Read the model definition and answer for the solid it produces. Units are mm, in the model's axes. Round coordinates to 2 decimals unless told otherwise and drop trailing zeros. Loops run counter-clockwise (first coordinate to the right, second up) from the corner with the lowest first, then second, coordinate; pieces in that order, holes last. Notation, with made-up numbers: M 69,-23.75 L 121,-23.75 A22 ccw 121,-14.75 Z; hole C 83.25,19 d9. An arc over 180 degrees is marked long. Answer as CSV lines item,"result".
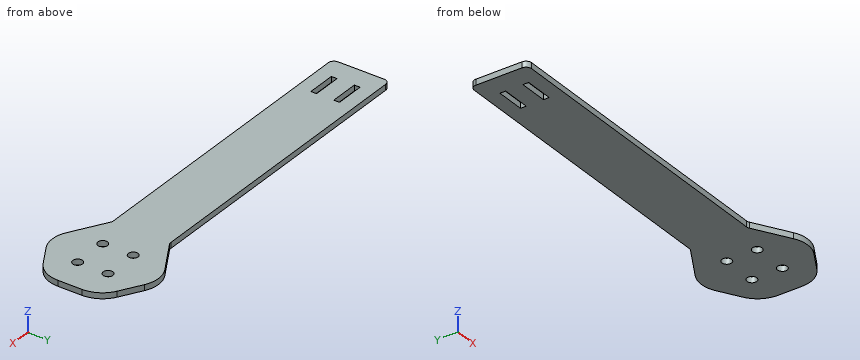
```python
from build123d import *

# Parameters (mm, degrees)
SKETCH1_W           = 107.330973451
SKETCH1_H           = 20
SKETCH1_W_2         = 10
SKETCH1_H_2         = 2
SKETCH1_R           = 12.25
SKETCH1_R_2         = 1.7
BOSS_EXTRUDE3_DEPTH = 2
FILLET5_R           = 10
FILLET6_R           = 10
FILLET7_R           = 10
FILLET8_R           = 10
FILLET14_R          = 2
FILLET15_R          = 2
FILLET16_R          = 2


with BuildPart() as part:
    # Sketch1 → Boss-Extrude3 (new body)
    # profile 1 of 4: a face of its own
    with BuildSketch(Plane.XY):
        with Locations((53.665486726, -20)):
            Rectangle(SKETCH1_W, SKETCH1_H)
        with Locations((12.5, -24)):
            Rectangle(SKETCH1_W_2, SKETCH1_H_2, mode=Mode.SUBTRACT)
        with Locations((12.5, -16)):
            Rectangle(SKETCH1_W_2, SKETCH1_H_2, mode=Mode.SUBTRACT)
    # profile 2 of 4: a face of its own
    with BuildSketch(Plane.XY):
        Polygon((140, -8.861471272), (124.651481526, 0), (107.330973451, -10), (107.330973451, -30), (124.651481526, -40), (140, -31.138528728), align=None)
        with Locations((124.651481526, -20)):
            Circle(SKETCH1_R, mode=Mode.SUBTRACT)
    # profile 3 of 4: a face of its own
    with BuildSketch(Plane.XY):
        with Locations((124.651481526, -20)):
            Circle(SKETCH1_R)
        with Locations((118.526481526, -25.304405598)):
            Circle(SKETCH1_R_2, mode=Mode.SUBTRACT)
        with Locations((130.776481526, -25.304405598)):
            Circle(SKETCH1_R_2, mode=Mode.SUBTRACT)
        with Locations((130.776481526, -14.695594402)):
            Circle(SKETCH1_R_2, mode=Mode.SUBTRACT)
        with Locations((118.526481526, -14.695594402)):
            Circle(SKETCH1_R_2, mode=Mode.SUBTRACT)
    # profile 4 of 4: a face of its own
    with BuildSketch(Plane.XY):
        Polygon((141.971989602, -10), (140, -8.861471272), (140, -31.138528728), (141.971989602, -30), align=None)
    extrude(amount=BOSS_EXTRUDE3_DEPTH)

    # Fillet5
    fillet5_edges = [part.edges().sort_by_distance(p)[0] for p in [
        (124.651481526, 0, 1),
    ]]
    fillet(fillet5_edges, radius=FILLET5_R)

    # Fillet6
    fillet6_edges = [part.edges().sort_by_distance(p)[0] for p in [
        (141.971989602, -10, 1),
    ]]
    fillet(fillet6_edges, radius=FILLET6_R)

    # Fillet7
    fillet7_edges = [part.edges().sort_by_distance(p)[0] for p in [
        (141.971989602, -30, 1),
    ]]
    fillet(fillet7_edges, radius=FILLET7_R)

    # Fillet8
    fillet8_edges = [part.edges().sort_by_distance(p)[0] for p in [
        (124.651481526, -40, 1),
    ]]
    fillet(fillet8_edges, radius=FILLET8_R)

    # Fillet14
    fillet14_edges = [part.edges().sort_by_distance(p)[0] for p in [
        (0, -30, 1),
        (0, -10, 1),
    ]]
    fillet(fillet14_edges, radius=FILLET14_R)

    # Fillet15
    fillet15_edges = [part.edges().sort_by_distance(p)[0] for p in [
        (107.330973451, -10, 1),
    ]]
    fillet(fillet15_edges, radius=FILLET15_R)

    # Fillet16
    fillet16_edges = [part.edges().sort_by_distance(p)[0] for p in [
        (107.330973451, -30, 1),
    ]]
    fillet(fillet16_edges, radius=FILLET16_R)


solid = part.part
```
1) Straight lines are drawn through the part: line 1 (Y direction, x = 15.5, z = 1.05); line 2 (X direction, y = -25.5, z = 0.6); line 3 (X direction, y = -23.5, z = 1.6). For each, find the intervals that lie inside material, in ascending order.
Evaluation:
line 1,"y = -30 to -25, -23 to -17, -15 to -10"
line 2,"x = 0 to 116.84, 120.22 to 129.09, 132.47 to 141.89"
line 3,"x = 0 to 7.5, 17.5 to 141.97"
2) Each of these flat-tipped pins is pushed along its axis until it touches: P1, Ø2, axis at x = 130.78, y = -25.3, coming from the +Z side; P2, Ø4, axis at x = 118.53, y = -14.7, coming from the -Z side; P3, Ø0.6, axis at x = 48.5, z = 0.5, coming from the +Y side; P4, Ø0.6, axis at x = 55.5, z = 1.5, coming from the -Y side. Where does it stop, or does it pass through?
Evaluation:
P1,"passes through"
P2,"stops at z = 0"
P3,"stops at y = -10"
P4,"stops at y = -30"
3) Find section B-B, the plane y = -5.5. Give the vertices of the cut face in (x, z), then the cut area to 3 significant figures.
Evaluation:
outline,"M 115.13,0 L 134.18,0 L 134.18,2 L 115.13,2 Z"
area,"38.1 mm^2"
4) Find section A-A, the plane x = 23.5. Give the vertices of the cut face in (y, z), then the cut area to 3 significant figures.
Evaluation:
outline,"M -30,0 L -10,0 L -10,2 L -30,2 Z"
area,"40.0 mm^2"
5) Find section C-C, the plane z = 0.8. Count the separate pieces of the cut face and the enclosed holes in it, then the cut area to 3 significant figures.
Evaluation:
separate pieces,"1"
enclosed holes,"6"
area,"3,090 mm^2"
